from build123d import *

# Parameters (mm, degrees)
SKETCH1_R           = 7.5
SKETCH1_R_2         = 1.6
SKETCH1_R_3         = 45
BOSS_EXTRUDE1_DEPTH = 65
SKETCH1_3_R         = 7.5
SKETCH1_3_R_2       = 1.6
BOSS_EXTRUDE2_DEPTH = 3.2
SKETCH1_5_R         = 1.6
SKETCH1_5_R_2       = 45
CUT_EXTRUDE2_DEPTH  = 55


with BuildPart() as part:
    # Sketch1 → Boss-Extrude1 (new body)
    with BuildSketch(Plane(origin=(0, 0, 0), x_dir=(1, 0, 0), z_dir=(0, 1, 0))):
        with BuildLine():
            Line((53.560713214, -12.5), (122.5, -12.5))
            ThreePointArc((122.5, -12.5), (135, 0), (122.5, 12.5))
            Line((122.5, 12.5), (53.560713214, 12.5))
            ThreePointArc((53.560713214, 12.5), (38.890872965, 38.890872965), (12.5, 53.560713214))
            Line((12.5, 53.560713214), (12.5, 122.5))
            ThreePointArc((12.5, 122.5), (0, 135), (-12.5, 122.5))
            Line((-12.5, 122.5), (-12.5, 53.560713214))
            ThreePointArc((-12.5, 53.560713214), (-38.890872965, 38.890872965), (-53.560713214, 12.5))
            Line((-53.560713214, 12.5), (-122.5, 12.5))
            ThreePointArc((-122.5, 12.5), (-135, 0), (-122.5, -12.5))
            Line((-122.5, -12.5), (-53.560713214, -12.5))
            ThreePointArc((-53.560713214, -12.5), (-38.890872965, -38.890872965), (-12.5, -53.560713214))
            Line((-12.5, -53.560713214), (-12.5, -122.5))
            ThreePointArc((-12.5, -122.5), (0, -135), (12.5, -122.5))
            Line((12.5, -122.5), (12.5, -53.560713214))
            ThreePointArc((12.5, -53.560713214), (38.890872965, -38.890872965), (53.560713214, -12.5))
        make_face()
        with Locations((122.5, 0)):
            Circle(SKETCH1_R, mode=Mode.SUBTRACT)
        with Locations((25, 43.301270189)):
            Circle(SKETCH1_R_2, mode=Mode.SUBTRACT)
        with Locations((0, 50)):
            Circle(SKETCH1_R_2, mode=Mode.SUBTRACT)
        with Locations((-25, -43.301270189)):
            Circle(SKETCH1_R_2, mode=Mode.SUBTRACT)
        with Locations((0, -50)):
            Circle(SKETCH1_R_2, mode=Mode.SUBTRACT)
        with Locations((-43.301270189, -25)):
            Circle(SKETCH1_R_2, mode=Mode.SUBTRACT)
        with Locations((25, -43.301270189)):
            Circle(SKETCH1_R_2, mode=Mode.SUBTRACT)
        with Locations((43.301270189, -25)):
            Circle(SKETCH1_R_2, mode=Mode.SUBTRACT)
        with Locations((50, 0)):
            Circle(SKETCH1_R_2, mode=Mode.SUBTRACT)
        with Locations((-50, 0)):
            Circle(SKETCH1_R_2, mode=Mode.SUBTRACT)
        with Locations((-43.301270189, 25)):
            Circle(SKETCH1_R_2, mode=Mode.SUBTRACT)
        Circle(SKETCH1_R_3, mode=Mode.SUBTRACT)
        with Locations((-25, 43.301270189)):
            Circle(SKETCH1_R_2, mode=Mode.SUBTRACT)
        with Locations((43.301270189, 25)):
            Circle(SKETCH1_R_2, mode=Mode.SUBTRACT)
        with Locations((0, 122.5)):
            Circle(SKETCH1_R, mode=Mode.SUBTRACT)
        with Locations((0, -122.5)):
            Circle(SKETCH1_R, mode=Mode.SUBTRACT)
        with Locations((-122.5, 0)):
            Circle(SKETCH1_R, mode=Mode.SUBTRACT)
    extrude(amount=BOSS_EXTRUDE1_DEPTH)

    # Sketch1<3> → Boss-Extrude2 (add)
    with BuildSketch(Plane(origin=(0, 0, 0), x_dir=(1, 0, 0), z_dir=(0, 1, 0))):
        with Locations((0, -122.5)):
            Circle(SKETCH1_3_R)
        with Locations((0, -122.5)):
            Circle(SKETCH1_3_R_2, mode=Mode.SUBTRACT)
        with Locations((122.5, 0)):
            Circle(SKETCH1_3_R)
        with Locations((122.5, 0)):
            Circle(SKETCH1_3_R_2, mode=Mode.SUBTRACT)
        with Locations((0, 122.5)):
            Circle(SKETCH1_3_R)
        with Locations((0, 122.5)):
            Circle(SKETCH1_3_R_2, mode=Mode.SUBTRACT)
        with Locations((-122.5, 0)):
            Circle(SKETCH1_3_R)
        with Locations((-122.5, 0)):
            Circle(SKETCH1_3_R_2, mode=Mode.SUBTRACT)
    extrude(amount=BOSS_EXTRUDE2_DEPTH)

    # Sketch1<5> → Cut-Extrude2 (cut)
    with BuildSketch(Plane(origin=(0, 0, 0), x_dir=(1, 0, 0), z_dir=(0, 1, 0))):
        with BuildLine():
            ThreePointArc((122.5, -12.5), (110, 0), (122.5, 12.5))
            Line((122.5, 12.5), (53.560713214, 12.5))
            ThreePointArc((53.560713214, 12.5), (38.890872965, 38.890872965), (12.5, 53.560713214))
            Line((12.5, 53.560713214), (12.5, 122.5))
            ThreePointArc((12.5, 122.5), (0, 110), (-12.5, 122.5))
            Line((-12.5, 122.5), (-12.5, 53.560713214))
            ThreePointArc((-12.5, 53.560713214), (-38.890872965, 38.890872965), (-53.560713214, 12.5))
            Line((-53.560713214, 12.5), (-122.5, 12.5))
            ThreePointArc((-122.5, 12.5), (-110, 0), (-122.5, -12.5))
            Line((-122.5, -12.5), (-53.560713214, -12.5))
            ThreePointArc((-53.560713214, -12.5), (-38.890872965, -38.890872965), (-12.5, -53.560713214))
            Line((-12.5, -53.560713214), (-12.5, -122.5))
            ThreePointArc((-12.5, -122.5), (0, -110), (12.5, -122.5))
            Line((12.5, -122.5), (12.5, -53.560713214))
            ThreePointArc((12.5, -53.560713214), (38.890872965, -38.890872965), (53.560713214, -12.5))
            Line((53.560713214, -12.5), (122.5, -12.5))
        make_face()
        with Locations((0, 50)):
            Circle(SKETCH1_5_R, mode=Mode.SUBTRACT)
        with Locations((25, 43.301270189)):
            Circle(SKETCH1_5_R, mode=Mode.SUBTRACT)
        with Locations((-25, -43.301270189)):
            Circle(SKETCH1_5_R, mode=Mode.SUBTRACT)
        with Locations((0, -50)):
            Circle(SKETCH1_5_R, mode=Mode.SUBTRACT)
        with Locations((-43.301270189, -25)):
            Circle(SKETCH1_5_R, mode=Mode.SUBTRACT)
        with Locations((25, -43.301270189)):
            Circle(SKETCH1_5_R, mode=Mode.SUBTRACT)
        with Locations((43.301270189, -25)):
            Circle(SKETCH1_5_R, mode=Mode.SUBTRACT)
        with Locations((50, 0)):
            Circle(SKETCH1_5_R, mode=Mode.SUBTRACT)
        with Locations((-50, 0)):
            Circle(SKETCH1_5_R, mode=Mode.SUBTRACT)
        with Locations((-43.301270189, 25)):
            Circle(SKETCH1_5_R, mode=Mode.SUBTRACT)
        Circle(SKETCH1_5_R_2, mode=Mode.SUBTRACT)
        with Locations((-25, 43.301270189)):
            Circle(SKETCH1_5_R, mode=Mode.SUBTRACT)
        with Locations((43.301270189, 25)):
            Circle(SKETCH1_5_R, mode=Mode.SUBTRACT)
    extrude(amount=CUT_EXTRUDE2_DEPTH, mode=Mode.SUBTRACT)


solid = part.part
The model under review builds one solid part; all positions refer to its coordinate system, in mm. A direction names the side the tool comes from. Round coordinates to 2 decimals unless told otherwise and drop trailing zeros. Write each loop counter-clockwise with the first axis right and the second up, starting at its lowest first coordinate (ties: lowest second). Pieces come first, ordered by that corner, then holes. Notation, with made-up numbers: (-23, 85.5) -> (4, 85.5) arc R15 cw to (4, 100.5) -> close; hole circle Ø7 at (-21.75, -18). An arc over 180 degrees is marked (long way). Answer as a JSON object with one key per item and string values.
1. Machinability: for faces 4 (the face through (-1.63, 33.67, 129.82)), 5 (the face through (89, 60, -12.5)), 6 (the face through (-12.5, 60, -89)), which of the approach directions +Z, -Z, +X, -X, +Y, -Y give a long, thin tool a straight path to every point of the face, cutting with its end or side? Answer none if there is none.
Results found:
{"face 4": "+Y", "face 5": "-Z, +X, +Y, -Y", "face 6": "-Z, -X, +Y, -Y"}
2. The part is to be moulded in two halves that separate along Z. For faces 1 (the face through (0, 0, -120)), 2 (the face through (-134.894, 32.045, 1.627)), 3 (the face through (-1.627, 32.045, -134.894)), say which applies: pulls with the +Z half, pulls with the -Z half, needs draft (parallel to the pull), parting line crosses it, or undercut.
Results found:
{"face 1": "needs draft", "face 2": "parting line crosses it", "face 3": "undercut"}
3. We need section C-C on y = 61.5. State how many separate pieces and enclosed holes the cut face has, and give its area (3 significant figures).
Results found:
{"separate pieces": "1", "enclosed holes": "17", "area": "10,100 mm^2"}
4. We need section D-D on x = -73. State the section outline as (y, z) points.
Results found:
{"outline": "(55, -12.5) -> (65, -12.5) -> (65, 12.5) -> (55, 12.5) -> close"}
5. We need section B-B on z = -96. State the section outline as (x, y) points.
Results found:
{"outline": "(-12.5, 55) -> (12.5, 55) -> (12.5, 65) -> (-12.5, 65) -> close"}
6. Clearance check with flat-ended pins moving along their axes: pin 1 (5 mm diameter, centred on y = 60.5, z = -77.5, fed in from +X); pin 2 (4.5 mm diameter, centred on x = -3.5, z = -121.5, fed in from +Y); pin 3 (5 mm diameter, centred on x = 81, y = 59.5, fed in from +Z). State where each tip first meets the part, or that it passes through.
Results found:
{"pin 1": "stops at x = 12.5", "pin 2": "stops at y = 3.2", "pin 3": "stops at z = 12.5"}
7. We need section A-A on y = 17. State the section outline as (x, z) points.
Results found:
{"outline": "circle Ø25 at (-122.5, 0); circle Ø25 at (0, -122.5); circle Ø25 at (0, 122.5); circle Ø25 at (122.5, 0); hole circle Ø15 at (-122.5, 0); hole circle Ø15 at (0, -122.5); hole circle Ø15 at (0, 122.5); hole circle Ø15 at (122.5, 0)"}
8. To check wall thickness, follow line 1 along Z through (x, y) = (0, 61); line 2 along X through (y, z) = (62.75, 25); line 3 along X through (y, z) = (60, -121.5). State the ranges of each line that lie inside material, in increasing order.
Results found:
{"line 1": "z = -135 to -130, -115 to -51.6, -48.4 to -45, 45 to 48.4, 51.6 to 115, 130 to 135", "line 2": "x = -48.99 to -44.9, -41.7 to -37.42, 37.42 to 41.7, 44.9 to 48.99", "line 3": "x = -12.5 to -7.43, 7.43 to 12.5"}
